Drawing for the job (mm, zero at the part's lowest x, y, z). A direction names the side the tool comes from. Coordinates: 2 decimals unless noted, no trailing zeros. Write each loop counter-clockwise with the first axis right and the second up, starting at its lowest first coordinate (ties: lowest second). Pieces come first, ordered by that corner, then holes. Notation, with made-up numbers: (-7.5, 27) -> (36.5, 27) arc R13 ccw to (36.5, 44) -> close; hole circle Ø8 at (60, 5). An arc over 180 degrees is marked (long way). Answer as CSV lines item,"result".
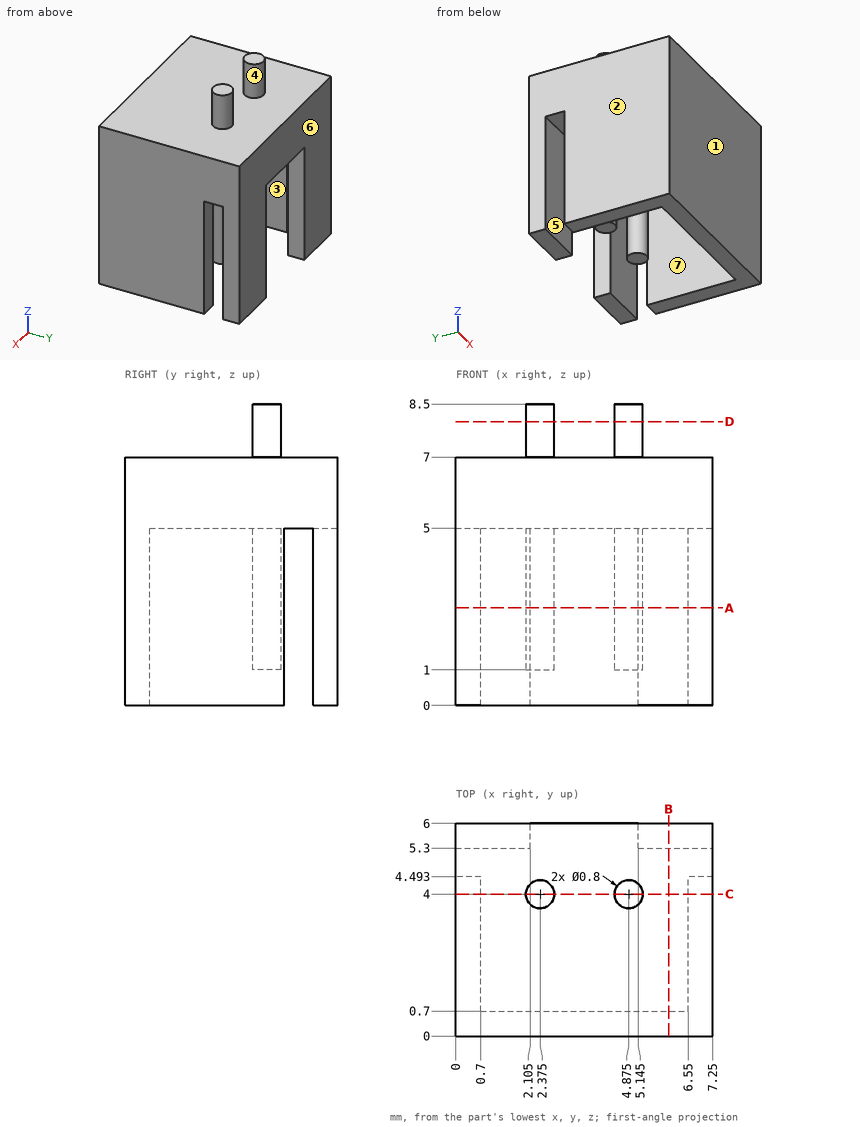
Item 1: Saw through at C-C on y = 4. Give the cut face in (x, z) (3 decimals), and give its area (3 significant figures).
Answer below:
outline,"(0, 0) -> (0.7, 0) -> (0.7, 5) -> (1.975, 5) -> (1.975, 1) -> (2.775, 1) -> (2.775, 5) -> (4.475, 5) -> (4.475, 1) -> (5.275, 1) -> (5.275, 5) -> (6.55, 5) -> (6.55, 0) -> (7.25, 0) -> (7.25, 7) -> (5.275, 7) -> (5.275, 8.5) -> (4.475, 8.5) -> (4.475, 7) -> (2.775, 7) -> (2.775, 8.5) -> (1.975, 8.5) -> (1.975, 7) -> (0, 7) -> close"
area,"30.3 mm2"
Item 2: Saw through at A-A on z = 2.75. Give the cut face in (x, y) (3 decimals).
Answer below:
outline,"(0, 0) -> (7.25, 0) -> (7.25, 4.493) -> (6.55, 4.493) -> (6.55, 0.7) -> (0.7, 0.7) -> (0.7, 4.493) -> (0, 4.493) -> close; (0, 5.3) -> (2.105, 5.3) -> (2.105, 6) -> (0, 6) -> close; circle Ø0.8 at (2.375, 4); circle Ø0.8 at (4.875, 4); (5.145, 5.3) -> (7.25, 5.3) -> (7.25, 6) -> (5.145, 6) -> close"
Item 3: Two-plate mould, pull along X, no slides. Class the marked faces 1, 2 and 3: pulls with the +X half, pulls with the -X half, needs draft (parallel to the pull), parting line crosses it, or undercut.
Answer below:
face 1,"needs draft"
face 2,"pulls with the -X half"
face 3,"undercut"
Item 4: Wall check: line 1 (X direction, y = 2, z = 4.75); line 2 (X direction, y = 4.05, z = 2.5); line 3 (Y direction, x = 6.25, z = 2.25). Give the ranges that are in metal, low to high. Write a range as from..to.
Answer below:
line 1,"x = 0..0.7, 6.55..7.25"
line 2,"x = 0..0.7, 1.98..2.77, 4.48..5.27, 6.55..7.25"
line 3,"y = 0..0.7, 5.3..6"
Item 5: Saw through at D-D on z = 8. Give the cut face in (x, y) (3 decimals).
Answer below:
outline,"circle Ø0.8 at (2.375, 4); circle Ø0.8 at (4.875, 4)"
Item 6: 3-axis set-ups, long thin cutter, end or side, ignore diameter. For the marked faces 4, 5, 6 and 7: which of +Z, -Z, +X, -X, +Y, -Y reach the whole face in a straight line?
Answer below:
face 4,"+Z"
face 5,"-Z, +X, -X"
face 6,"+Z, -Z, +X, -X, +Y"
face 7,"-Z"
Item 7: Flat gauge pins, fed straight in: pin 1 (2.5 mm diameter, centred on x = 3.5, z = 2.5, fed in from +Y); pin 2 (1 mm diameter, centred on x = 2.5, y = 3.5, fed in from -Z). Where does each tip first touch, or does it go through?
Answer below:
pin 1,"stops at y = 4.4"
pin 2,"stops at z = 1"
Item 8: Saw through at B-B on x = 6. Give the cut face in (y, z), and give its area (3 significant figures).
Answer below:
outline,"(0, 0) -> (0.7, 0) -> (0.7, 5) -> (5.3, 5) -> (5.3, 0) -> (6, 0) -> (6, 7) -> (0, 7) -> close"
area,"19.0 mm2"
